Work out the finished part from the listing and answer in its coordinate system (mm). Face numbers are marked on the shaded views. A direction names the side the tool comes from. Coordinates: 2 decimals unless noted, no trailing zeros. Order: outer loops, then holes, each group sorted by start corner. A loop starts at its lowest first (then second) coordinate and runs counter-clockwise, first axis right, second up. Notation, with made-up numbers: M -16,60 L -2,60 A25 ccw -2,96 Z; hole C 74.5,-22 d8. An arc over 180 degrees is marked long. Use a Markdown table: item, result.
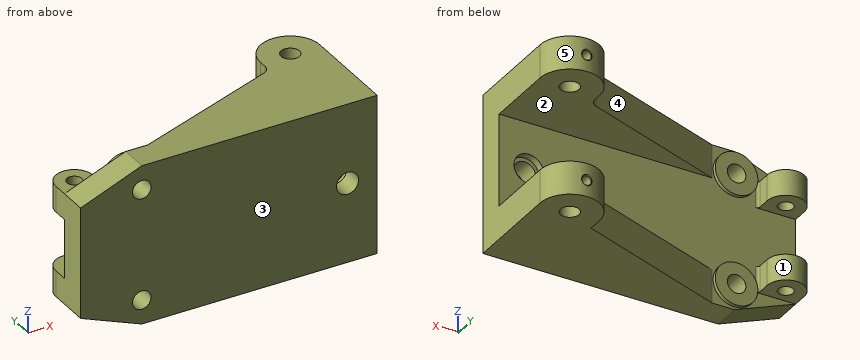
from build123d import *

# Parameters (mm, degrees)
BOSS_EXTRU_1_DEPTH           = 15
BOSS_EXTRU_2_DEPTH           = 18
BOSS_EXTRU_3_DEPTH           = 14
CONG_1_R                     = 5
ENL_V_MAT_EXTRU_1_DEPTH      = 189.917971617
ENL_V_MAT_EXTRU_1_DEPTH_BACK = 189.917971617
ESQUISSE4_R                  = 4
ENL_V_MAT_EXTRU_2_DEPTH      = 195.311605418
ENL_V_MAT_EXTRU_2_DEPTH_BACK = 195.311605418
ESQUISSE5_R                  = 5
ENL_V_MAT_EXTRU_3_DEPTH      = 175.255559452
ENL_V_MAT_EXTRU_3_DEPTH_BACK = 175.255559452
ESQUISSE6_R                  = 5.987648709
ESQUISSE7_R                  = 8
ENL_V_MAT_EXTRU_4_DEPTH      = 4
ENL_V_MAT_EXTRU_5_REACH      = 176.256
ESQUISSE12_R                 = 5
BOSS_EXTRU_4_START           = 2
ESQUISSE13_R                 = 11.5
ESQUISSE13_R_2               = 5
BOSS_EXTRU_4_DEPTH           = 2
CONG_2_R                     = 1.5


# Read off the part's stored shape, not the designer's step: Trou taraudé M61
with BuildPart() as part:
    # Esquisse1 → Boss.-Extru.1 (new body)
    with BuildSketch(Plane(origin=(0, 0, 0), x_dir=(1, 0, 0), z_dir=(0, 1, 0))):
        Polygon((0, -43), (-127, -43), (-160, -30), (-160, 0), (0, 0), align=None)
    boss_extru_1 = extrude(amount=BOSS_EXTRU_1_DEPTH)

    # Esquisse2 → Boss.-Extru.2 (add)
    with BuildSketch(Plane.XY.offset(43)):
        with BuildLine():
            Line((-32, 45.209529444), (-32, 53))
            ThreePointArc((-32, 53), (-16, 69), (0, 53))
            Line((0, 53), (0, 15))
            Line((0, 15), (-115, 15))
            Line((-115, 15), (-32, 45.209529444))
        make_face()
    boss_extru_2 = extrude(amount=-BOSS_EXTRU_2_DEPTH)

    # Esquisse3 → Boss.-Extru.3 (add)
    with BuildSketch(Plane.XY.offset(30)):
        with BuildLine():
            Line((-140, 23), (-140, 15))
            Line((-140, 15), (-160, 15))
            Line((-160, 15), (-160, 23))
            ThreePointArc((-160, 23), (-150, 33), (-140, 23))
        make_face()
    boss_extru_3 = extrude(amount=-BOSS_EXTRU_3_DEPTH)

    # Congé1
    cong_1_edges = [part.edges().sort_by_distance(p)[0] for p in [
        (-32, 45.209529444, 34),
    ]]
    fillet(cong_1_edges, radius=CONG_1_R)

    # Symétrie1: Boss.-Extru.1, Boss.-Extru.2, Boss.-Extru.3 across plane
    add(boss_extru_1.mirror(Plane.XY))
    add(boss_extru_2.mirror(Plane.XY))
    add(boss_extru_3.mirror(Plane.XY))

    # Esquisse4 → Enlèv. mat.-Extru.1 (cut, two sides: drawn at the far end of the back side and taken through both)
    with BuildSketch(Plane.XY.offset(30).offset(-ENL_V_MAT_EXTRU_1_DEPTH_BACK)):
        with Locations(Location((-150, 23, 0), (0, 0, 180))):
            Circle(ESQUISSE4_R)
    extrude(amount=ENL_V_MAT_EXTRU_1_DEPTH + ENL_V_MAT_EXTRU_1_DEPTH_BACK, mode=Mode.SUBTRACT)

    # Esquisse5 → Enlèv. mat.-Extru.2 (cut, two sides: drawn at the far end of the back side and taken through both)
    with BuildSketch(Plane.XY.offset(43).offset(-ENL_V_MAT_EXTRU_2_DEPTH_BACK)):
        with Locations((-16, 53)):
            Circle(ESQUISSE5_R)
    extrude(amount=ENL_V_MAT_EXTRU_2_DEPTH + ENL_V_MAT_EXTRU_2_DEPTH_BACK, mode=Mode.SUBTRACT)

    # Esquisse6 → Enlèv. mat.-Extru.3 (cut, two sides: drawn at the far end of the back side and taken through both)
    with BuildSketch(Plane(origin=(0, 15, 0), x_dir=(1, 0, 0), z_dir=(0, 1, 0)).offset(-ENL_V_MAT_EXTRU_3_DEPTH_BACK)):
        with Locations(Location((-16, 0, 0), (0, 0, 270))):
            Circle(ESQUISSE6_R)
    extrude(amount=ENL_V_MAT_EXTRU_3_DEPTH + ENL_V_MAT_EXTRU_3_DEPTH_BACK, mode=Mode.SUBTRACT)

    # Esquisse7 → Enlèv. mat.-Extru.4 (cut)
    with BuildSketch(Plane(origin=(0, 15, 0), x_dir=(1, 0, 0), z_dir=(0, 1, 0))):
        with Locations(Location((-16, 0, 0), (0, 0, 270))):
            Circle(ESQUISSE7_R)
    extrude(amount=-ENL_V_MAT_EXTRU_4_DEPTH, mode=Mode.SUBTRACT)

    # Trou taraudé M61 outline → Trou taraudé M61 (revolve, cut)
    with BuildSketch(Plane(origin=(-16, 0, 34), x_dir=(1, 0, 0), z_dir=(0, 0, 1))):
        Polygon((0, 57.329808988), (2.5, 57.329808988), (2.5, 68.475), (3.02508907, 69.00008907), (0, 69.00008907), align=None)
    revolve(axis=Axis((-16, 0, 34), (0, 1, 0)), mode=Mode.SUBTRACT)

    # Trou taraud_ M61 2 outline → Trou taraud_ M61 2 (revolve, cut)
    with BuildSketch(Plane(origin=(-16, 0, -34), x_dir=(1, 0, 0), z_dir=(0, 0, 1))):
        Polygon((3.025080927, 69.000080927), (0, 69.000080927), (0, 57.329808988), (2.5, 57.329808988), (2.5, 68.475), align=None)
    revolve(axis=Axis((-16, 0, -34), (0, 1, 0)), mode=Mode.SUBTRACT)

    # Esquisse12 → Enlèv. mat.-Extru.5 (cut, up to next)
    with BuildSketch(Plane(origin=(0, 15, 0), x_dir=(1, 0, 0), z_dir=(0, 1, 0)), mode=Mode.PRIVATE) as enl_v_mat_extru_5_sk1:
        with Locations(Location((-127, -30, 0), (0, 0, 270))):
            Circle(ESQUISSE12_R)
    enl_v_mat_extru_5_tool1 = extrude(enl_v_mat_extru_5_sk1.sketch, amount=-ENL_V_MAT_EXTRU_5_REACH, mode=Mode.PRIVATE) & part.part
    # Esquisse12 → Enlèv. mat.-Extru.5 (cut, up to next)
    with BuildSketch(Plane(origin=(0, 15, 0), x_dir=(1, 0, 0), z_dir=(0, 1, 0)), mode=Mode.PRIVATE) as enl_v_mat_extru_5_sk2:
        with Locations(Location((-127, 30, 0), (0, 0, 270))):
            Circle(ESQUISSE12_R)
    enl_v_mat_extru_5_tool2 = extrude(enl_v_mat_extru_5_sk2.sketch, amount=-ENL_V_MAT_EXTRU_5_REACH, mode=Mode.PRIVATE) & part.part
    add(enl_v_mat_extru_5_tool1.solids().sort_by_distance((-127, 15, 30))[0], mode=Mode.SUBTRACT)
    add(enl_v_mat_extru_5_tool2.solids().sort_by_distance((-127, 15, -30))[0], mode=Mode.SUBTRACT)

    # Esquisse13 → Boss.-Extru.4 (add)
    # profile 1 of 2: a face of its own
    with BuildSketch(Plane(origin=(0, 15, 0), x_dir=(1, 0, 0), z_dir=(0, 1, 0)).offset(BOSS_EXTRU_4_START)):
        with Locations(Location((-127, -30, 0), (0, 0, 90))):
            Circle(ESQUISSE13_R)
        with Locations(Location((-127, -30, 0), (0, 0, 270))):
            Circle(ESQUISSE13_R_2, mode=Mode.SUBTRACT)
    # profile 2 of 2: a face of its own
    with BuildSketch(Plane(origin=(0, 15, 0), x_dir=(1, 0, 0), z_dir=(0, 1, 0)).offset(BOSS_EXTRU_4_START)):
        with Locations(Location((-127, 30, 0), (0, 0, 90))):
            Circle(ESQUISSE13_R)
        with Locations(Location((-127, 30, 0), (0, 0, 270))):
            Circle(ESQUISSE13_R_2, mode=Mode.SUBTRACT)
    extrude(amount=-BOSS_EXTRU_4_DEPTH)

    # Congé2
    cong_2_edges = [part.edges().sort_by_distance(p)[0] for p in [
        (-140, 15, 23),
        (-140, 15, -23),
    ]]
    fillet(cong_2_edges, radius=CONG_2_R - 0.0001)  # a hair under: the kernel refuses the full size


solid = part.part
(1) Given P1, Ø7, axis at x = -123.5, z = -33.5, coming from the +Y side; P2, Ø4.5, axis at x = -16, z = -34, coming from the +Y side; P3, Ø20, axis at x = -154, y = 22.5, coming from the -Z side, each flat-ended and moving along its own axis, determine where each tip first touches the part or whether it passes through.
Conclusion:
| item | result |
|---|---|
| P1 | y = 17 |
| P2 | y = 48.53 |
| P3 | z = -34.97 |
(2) A cutting plane is placed at C-C (x = -107.5). Determine the outline of the cut face in (y, z).
Conclusion:
| item | result |
|---|---|
| outline | M 0,-43 L 17.73,-43 L 17.73,-25 L 15,-25 L 15,25 L 17.73,25 L 17.73,43 L 0,43 Z |
(3) A cutting plane is placed at B-B (y = 31). Determine the outline of the cut face in (x, z).
Conclusion:
| item | result |
|---|---|
| outline | M -156,-30 L -144,-30 L -144,-16 L -156,-16 Z; M -156,16 L -144,16 L -144,30 L -156,30 Z; M -71.04,-43 L 0,-43 L 0,-25 L -71.04,-25 Z; M -71.04,25 L 0,25 L 0,43 L -71.04,43 Z |
(4) Straight lines are drawn through the part: L1, parallel to Z at x = -17.5, y = 46.5; L2, parallel to Z at x = -16, y = 60.75; L3, parallel to Y at x = -149.5, z = 27.5. For each, find the intervals that lie inside material, in ascending order.
Conclusion:
| item | result |
|---|---|
| L1 | -43 to -25, 25 to 43 |
| L2 | -43 to -36.5, -31.5 to -25, 25 to 31.5, 36.5 to 43 |
| L3 | 0 to 19.03, 26.97 to 32.99 |
(5) A cutting plane is placed at D-D (x = -143.5). Determine the outline of the cut face in (y, z), then the cut area to 3 significant figures.
Conclusion:
| item | result |
|---|---|
| outline | M 0,-36.5 L 15,-36.5 L 15,-30 L 30.6,-30 L 30.6,-16 L 15,-16 L 15,16 L 30.6,16 L 30.6,30 L 15,30 L 15,36.5 L 0,36.5 Z |
| area | 1,530 mm2 |
(6) Which of the six approach directions +Z, -Z, +X, -X, +Y, -Y give full straight-line access (tool end or side, diameter ignored) to the marked faces 1 and 2?
Conclusion:
| item | result |
|---|---|
| face 1 | +Z, -Z, +Y |
| face 2 | +X, +Y |
(7) Determine the mould class of the marked faces 3, 4 and 5 for opening direction X: pulls with the +X half, pulls with the -X half, needs draft (parallel to the pull), parting line crosses it, or undercut.
Conclusion:
| item | result |
|---|---|
| face 3 | needs draft |
| face 4 | undercut |
| face 5 | parting line crosses it |
(8) A cutting plane is placed at A-A (z = 0). Determine the outline of the cut face in (x, y), then the cut area to 3 significant figures.
Conclusion:
| item | result |
|---|---|
| outline | M -160,0 L -21.99,0 L -21.99,11 L -24,11 L -24,15 L -160,15 Z; M -10.01,0 L 0,0 L 0,15 L -8,15 L -8,11 L -10.01,11 Z |
| area | 2,200 mm2 |
